from build123d import *

# Parameters (mm, degrees)
SKETCH1_W           = 465
SKETCH1_H           = 90
SKETCH1_R           = 2.55
BOSS_EXTRUDE1_DEPTH = 2.2479
SKETCH5_W           = 118
SKETCH5_H           = 70
CUT_EXTRUDE2_DEPTH  = 237.85747237
SKETCH7_R           = 2.55
CUT_EXTRUDE3_DEPTH  = 4.4958


with BuildPart() as part:
    # Sketch1 → Boss-Extrude1 (new, symmetric)
    with BuildSketch(Plane.XY):
        Rectangle(SKETCH1_W, SKETCH1_H)
        with Locations((-222.5, 35)):
            Circle(SKETCH1_R, mode=Mode.SUBTRACT)
        with Locations((-222.5, -35)):
            Circle(SKETCH1_R, mode=Mode.SUBTRACT)
        with Locations((0, 35)):
            Circle(SKETCH1_R, mode=Mode.SUBTRACT)
        with Locations((-114.975, 35)):
            Circle(SKETCH1_R, mode=Mode.SUBTRACT)
        with Locations(Location((222.5, -35, 0), (0, 0, 180))):
            Circle(SKETCH1_R, mode=Mode.SUBTRACT)
        with Locations(Location((222.5, 35, 0), (0, 0, 180))):
            Circle(SKETCH1_R, mode=Mode.SUBTRACT)
        with Locations(Location((114.975, 35, 0), (0, 0, 180))):
            Circle(SKETCH1_R, mode=Mode.SUBTRACT)
    extrude(amount=BOSS_EXTRUDE1_DEPTH, both=True)

    # Sketch5 → Cut-Extrude2 (cut, through all)
    with BuildSketch(Plane(origin=(0, 0, -2.2479), x_dir=(-1, 0, 0), z_dir=(0, 0, -1))):
        with Locations((153.5, -10)):
            Rectangle(SKETCH5_W, SKETCH5_H)
    extrude(amount=-CUT_EXTRUDE2_DEPTH, mode=Mode.SUBTRACT)

    # Sketch7 → Cut-Extrude3 (cut)
    with BuildSketch(Plane(origin=(0, 0, -2.2479), x_dir=(-1, 0, 0), z_dir=(0, 0, -1))):
        with Locations((84.8, -30)):
            Circle(SKETCH7_R)
    extrude(amount=-CUT_EXTRUDE3_DEPTH, mode=Mode.SUBTRACT)


solid = part.part
Geometry: final body of the model. Coordinates: model frame, mm. Round coordinates to 2 decimals unless told otherwise and drop trailing zeros. Loops run counter-clockwise (first coordinate to the right, second up) from the corner with the lowest first, then second, coordinate; pieces in that order, holes last.
Q1. Section A-A on y = 9.5. Return loops of the section in (x, z), plus the area to 3 significant figures.
Q2. Material intervals for L1, parallel to Y at x = 222.5, z = 0.1; L2, parallel to X at y = -34.5, z = -1.9; L3, parallel to X at y = -16.5, z = 0, sorted ascending.
Q3. Section B-B on z = 0.2. State how many separate pieces and enclosed holes the cut face has, plus the area to 3 significant figures.
Q4. Pin query (flat end, axial travel): P1, Ø1.3, axis at x = -154, z = 0.5, coming from the -Y side. Return the tip coordinate at first contact, or that it passes through.
Q5. Section C-C on x = -124. Return loops of the section in (y, z), plus the area to 3 significant figures.
Evaluation:
1. outline: (-232.5, -2.25) - (-212.5, -2.25) - (-212.5, 2.25) - (-232.5, 2.25) - close; (-94.5, -2.25) - (232.5, -2.25) - (232.5, 2.25) - (-94.5, 2.25) - close
1. area: 1,560 mm2
2. L1: y = -45 to -37.55, -32.45 to 32.45, 37.55 to 45
2. L2: x = -232.5 to -225, -220 to -212.5, -94.5 to 220, 225 to 232.5
2. L3: x = -232.5 to -212.5, -94.5 to 232.5
3. separate pieces: 1
3. enclosed holes: 8
3. area: 33,400 mm2
4. P1: stops at y = 25
5. outline: (25, -2.25) - (45, -2.25) - (45, 2.25) - (25, 2.25) - close
5. area: 89.9 mm2
